Check sheet for the modelled part. Datum: model origin and axes. Units: mm. Face numbers are marked on the shaded views. A direction names the side the tool comes from. Give positions to 0.01 mm unless a question says otherwise; leave off trailing zeros. Write each loop counter-clockwise with the first axis right and the second up, starting at its lowest first coordinate (ties: lowest second). Pieces come first, ordered by that corner, then holes. Notation, with made-up numbers: M 67,69.5 L 92,69.5 A29 ccw 92,100.5 Z; hole C 55,-6 d4. An arc over 180 degrees is marked long. Write item = value, one per line. Start each with the question number.
1) Sectioned sample at D-D, the plane x = -5.5. Record the cut outline in (y, z), then the cut area to 3 significant figures.
2) Sectioned sample at B-B, the plane y = 6. Record the cut outline in (x, z), then the cut area to 3 significant figures.
3) Sectioned sample at C-C, the plane z = -65.5. Count the separate pieces of the cut face and the enclosed holes in it, then the cut area to 3 significant figures.
4) Set-up check for the marked faces 1, 2, 3 and 4: record each of +Z, -Z, +X, -X, +Y, -Y from which the full face is reachable in a straight line by a thin tool's end or side.
5) Scan lines: L1, parallel to X at y = -100.5, z = -83; L2, parallel to X at y = -56.5, z = -37; L3, parallel to Y at x = 57, z = -51. Record each from-to range of solid material in increasing order.
6) Draft check along X on the marked faces 5, 6 and 7. Enter one of: pulls with the +X half, pulls with the -X half, needs draft (parallel to the pull), parting line crosses it, or undercut.
7) Gauge pin test, flat ends, axial feed: pin 1 (2 mm diameter, centred on y = -12.5, z = -41.5, fed in from +X); pin 2 (5 mm diameter, centred on y = 17.5, z = -37, fed in from +X); pin 3 (12 mm diameter, centred on x = 28.5, z = -89.5, fed in from +Y). Record the tip position at first contact, or that the pin passes through.
8) Sectioned sample at A-A, the plane x = -63. Record the cut outline in (y, z).
from build123d import *

# Parameters (mm, degrees)
F4_DEPTH = 100
F5_DEPTH = 100
F7_DEPTH = 25
F8_R     = 18.5
F9_DEPTH = 25


with BuildPart() as f4:
    # F0 (on Top) → F4 (new body)
    with BuildSketch(Plane.XY):
        Polygon((-100, -25), (25, -25), (95.7106781187, 45.7106781187), (70.7106781187, 70.7106781187), (0, 0), (-100, 0), align=None)
    extrude(amount=-F4_DEPTH)

    # F3 (on 3pt) → F5 (join)
    with BuildSketch(Plane(origin=(0, 0, 0), x_dir=(0.7071067812, -0.7071067812, 0), z_dir=(-0.7071067812, -0.7071067812, 0))):
        Polygon((0, 0), (0, -30), (51.9615242271, -30), (171.7339375866, -99.1506350946), (184.2339375866, -77.5), (50, 0), align=None)
    extrude(amount=-F5_DEPTH)

    # F6 (on face) → F7 (cut, through all)
    with BuildSketch(Plane.XZ.offset(25)):
        with BuildLine():
            Line((-50, -25), (-100, -25))
            Line((-100, -25), (-100, -75))
            Line((-100, -75), (-50, -75))
            ThreePointArc((-50, -75), (-25, -50), (-50, -25))
        make_face()
    extrude(amount=-F7_DEPTH, mode=Mode.SUBTRACT)

    # F8 (on face) → F9 (cut, through all)
    with BuildSketch(Plane(origin=(8.8388347648, -8.8388347648, 21.6506350946), x_dir=(0.9354143467, 0.133630621, -0.3273268354), z_dir=(0.3535533906, -0.3535533906, 0.8660254038))):
        with Locations((91.0206222635, -28.7252999487)):
            Circle(F8_R)
        with BuildLine():
            Line((112.710926197, -91.9592363695), (148.7168780859, -133.5353284006))
            Line((148.7168780859, -133.5353284006), (186.5133253868, -100.8026448652))
            Line((186.5133253868, -100.8026448652), (150.5073734979, -59.2265528341))
            ThreePointArc((150.5073734979, -59.2265528341), (115.2428080797, -56.6946709514), (112.710926197, -91.9592363695))
        make_face()
    extrude(amount=-F9_DEPTH, mode=Mode.SUBTRACT)


solid = f4.part
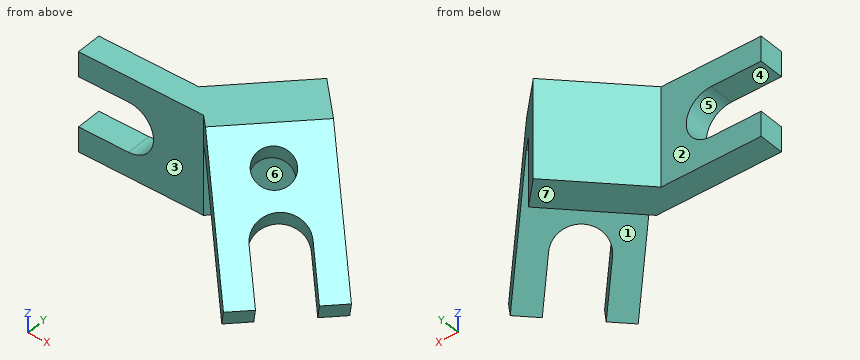
Data:
q1.outline = M -25,-100 L 0,-100 L 0,0 L -25,0 Z
q1.area = 2,500 mm2
q2.outline = M 6,-100 L 56,-100 L 56,-30 L 79.48,-30 L 135.42,-52.84 L 135.42,-23.97 L 76.71,0 L 6,0 Z
q2.area = 7,320 mm2
q3.separate_pieces = 3
q3.enclosed_holes = 0
q3.area = 7,140 mm2
q4.face_1 = -Z
q4.face_2 = +Z, -Z, -X, +Y
q4.face_3 = +Z, -Z, -X, -Y
q4.face_4 = -X, +Y, -Y
q5.L1 = 102.81 to 135.86
q5.L2 = 56.5 to 104.84
q5.L3 = 7 to 57
q6.face_5 = pulls with the -X half
q6.face_6 = undercut
q6.face_7 = needs draft
q7.pin_1 = 154.92
q7.pin_2 = 126.42
q7.pin_3 = 34.5
q8.outline = M -25,-100 L 0,-100 L 0,-75 L -25,-75 Z; M -25,-25 L 0,-25 L 0,0 L -25,0 Z
